For this review, take the finished solid that the model builds, in its own axes (mm). A direction names the side the tool comes from. Give positions to 0.01 mm unless a question says otherwise; leave off trailing zeros. Loops run counter-clockwise (first coordinate to the right, second up) from the corner with the lowest first, then second, coordinate; pieces in that order, holes last. Notation, with made-up numbers: (33.25, -29.5) -> (49.25, -29.5) arc R22 ccw to (49.25, -14.5) -> close; hole circle Ø10 at (14, 54.25). An arc over 180 degrees is marked (long way). One line per question, with ' | ' between items. Start each with the question number.
(1) Draft analysis for pull direction Z (two halves, no side actions). For faces 1 (the cylindrical face through (-0.69, 8, -3.1)), 2 (the flat face through (0.644, 8.264, 1.095)), 3 (the flat face through (0, 7.62, 2.1)), state which applies: +Z half, -Z half, draft (parallel to the pull), parting line (faces both ways), or undercut.
(2) Wall thickness on probe 1 along Y at (x, z) = (0.25, 2.5); probe 2 along Y at (x, z) = (0.75, -0.75); probe 3 along Z at (x, y) = (-2, 8): over which ranges is each line inside the solid? List them lowest first.
(3) Consider section B-B (y = 0.75). Write out the cut boundary in (x, z) (3 decimals).
(4) Tool access review of faces 4 (the cylindrical face through (0.41, 4.01, 1.86)), 5 (the flat face through (-1.27, 8, 0)), 6 (the flat face through (1.1, 8.89, 1.1)): name each direction out of +Z, -Z, +X, -X, +Y, -Y from which nothing blocks a thin tool from reaching the whole face with its end or side.
(5) Insertion check: P1, Ø1.5, axis at y = 3.5, z = 0, coming from the +X side (3 decimals); P2, Ø1, axis at y = 1, z = -1.5, coming from the +X side; P3, Ø1, axis at y = 4, z = 1.5, coming from the -X side. Each pin has a flat end and moves straight along its axis. Give the tip position at first contact, or say it passes through.
(6) Consider section A-A (z = 0). Write out the cut boundary in (x, y) (3 decimals), and give its area (3 significant figures).
Autodesk Inventor part; units mm, degrees
ref_plane "YZ Plane" through (0, 0, 0) normal (1, 0, 0) x (0, 1, 0)
ref_plane "XZ Plane" through (0, 0, 0) normal (0, 1, 0) x (-1, 0, 0)
ref_plane "XY Plane" through (0, 0, 0) normal (0, 0, 1) x (1, 0, 0)
sketch "Sketch1" plane through (0, 0, 0) normal (0, 1, 0) x (-1, 0, 0)
  point P0 (0, 0)
sketch "Sketch2" plane through (0, 0, 0) normal (0, 1, 0) x (-1, 0, 0)
  circle A0 centre (0, 0) radius 1.905
  dimension "d0" = 3.81
extrude "Extrusion1" add sketch "Sketch2" along normal blind 7.62
chamfer "Chamfer1" distance 0.508 angle 45 1 edges at (1.905, 0, 0)
sketch "Sketch3" plane through (0, 7.62, 0) normal (0, 1, 0) x (1, 0, 0)
  circle A0 centre (0, 0) radius 3.175
  dimension "d6" = 6.35
extrude "Extrusion2" add sketch "Sketch3" along normal blind 1.27
chamfer "Chamfer2" distance 0.508 angle 45 1 edges at (-3.175, 8.89, 0)
thread "Thread1"
sketch "Sketch4" plane through (0, 8.89, 0) normal (0, 1, 0) x (1, 0, 0)
  line L0 (0, -1.4665) -> (-1.27, -0.7332)
  line L1 (-1.27, -0.7332) -> (-1.27, 0.7332)
  line L2 (-1.27, 0.7332) -> (0, 1.4665)
  line L3 (0, 1.4665) -> (1.27, 0.7332)
  line L4 (1.27, 0.7332) -> (1.27, -0.7332)
  line L5 (1.27, -0.7332) -> (0, -1.4665)
  point P0 (0, 0)
  point P1 (0, 0)
  dimension "d14" = 2.54
extrude "Extrusion3" cut sketch "Sketch4" against normal blind 1.27
properties part number "Train_003_PracticeBolt" material "Stainless Steel"
A:
1) face 1: parting line | face 2: undercut | face 3: draft
2) probe 1: y = 7.62 to 8.89 | probe 2: y = 0 to 7.62 | probe 3: z = -2.47 to 2.47
3) outline: circle Ø3.81 at (0, 0)
4) face 4: -Y | face 5: +Y | face 6: +Z, -Z, +X, -X, +Y
5) P1: stops at x = 1.905 | P2: stops at x = 1.62 | P3: stops at x = -1.62
6) outline: (-3.175, 7.62) -> (-1.905, 7.62) -> (-1.905, 0.508) -> (-1.397, 0) -> (1.397, 0) -> (1.905, 0.508) -> (1.905, 7.62) -> (3.175, 7.62) -> (3.175, 8.382) -> (2.667, 8.89) -> (1.27, 8.89) -> (1.27, 7.62) -> (-1.27, 7.62) -> (-1.27, 8.89) -> (-2.667, 8.89) -> (-3.175, 8.382) -> close | area: 33.4 mm^2
